Geometry: see drawing. Coordinates: mm, zero at the bounding-box minimum. Round coordinates to 2 decimals unless told otherwise and drop trailing zeros. Order: outer loops, then holes, each group sorted by start corner. A loop starts at its lowest first (then second) coordinate and runs counter-clockwise, first axis right, second up.
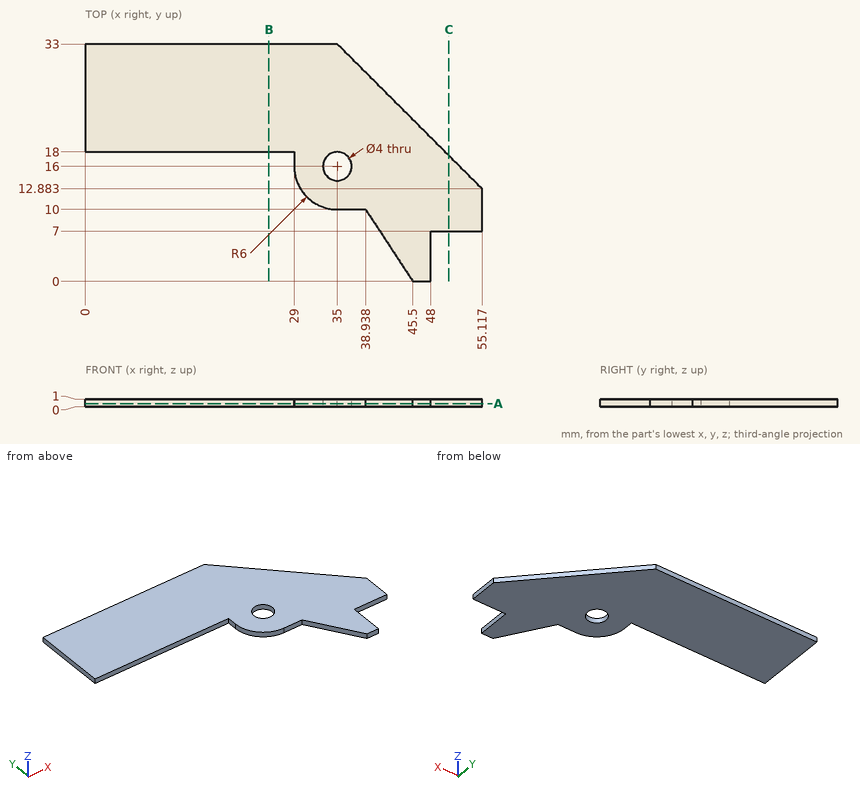
1. Section C-C on x = 50.5. Return loops of the section in (y, z).
2. Line query: line 1 along Y through (x, z) = (35, 0.6); line 2 along Y through (x, z) = (19, 0.75); line 3 along X through (y, z) = (28.5, 0.8). Output: solid intervals per line, ascending.
3. Section A-A on z = 0.4. Return loops of the section in (x, y).
4. First-contact query: pin 1 (0.5 mm diameter, centred on x = 36.5, z = 0.5, fed in from -Y). Flat tip, straight axial feed; report the tip coordinate or a pass-through.
5. Section B-B on x = 25.5. Return loops of the section in (y, z), plus the area to 3 significant figures.
Result:
1. outline: (7, 0) - (17.5, 0) - (17.5, 1) - (7, 1) - close
2. line 1: y = 10 to 14, 18 to 33
2. line 2: y = 18 to 33
2. line 3: x = 0 to 39.5
3. outline: (0, 18) - (29, 18) - (29, 16) arc R6 ccw to (35, 10) - (38.94, 10) - (45.5, 0) - (48, 0) - (48, 7) - (55.12, 7) - (55.12, 12.88) - (35, 33) - (0, 33) - close; hole circle Ø4 at (35, 16)
4. pin 1: stops at y = 10
5. outline: (18, 0) - (33, 0) - (33, 1) - (18, 1) - close
5. area: 15.0 mm2
